Build history of the part. All positions in model axes, mm. A direction names the side the tool comes from. Round coordinates to 2 decimals unless told otherwise and drop trailing zeros. Order: outer loops, then holes, each group sorted by start corner. A loop starts at its lowest first (then second) coordinate and runs counter-clockwise, first axis right, second up. Notation, with made-up numbers: (57, 6) - (100, 6) arc R22 cw to (100, 19) - close; hole circle Ø4 at (23.25, -5.75). An arc over 180 degrees is marked (long way). Write each question's results on one line, items separated by ' | '. Start each with the question number.
```python
from build123d import *

# Parameters (mm, degrees)
F1_DEPTH = 0.889


with BuildPart() as f1:
    # F0 (on Front) → F1 (new body)
    with BuildSketch(Plane.XZ):
        Polygon((-7.766421, 2.049147), (-9.697749, 3.149271), (-8.251928, 3.717801), (-8.401837, 4.58542), (-9.168207, 5.237091), (-10.238115, 4.58542), (-10.238115, 5.944121), (-7.570077, 7.6432), (-7.442288, 8.765532), (-8.34682, 9.053338), (-10.238115, 7.696539), (-10.238115, 10.554039), (-11.1125, 11.030715), (-12.026622, 10.656827), (-12.026622, 7.737654), (-13.897186, 9.053338), (-14.801892, 8.683302), (-14.616874, 7.614309), (-11.972634, 5.904664), (-11.972634, 4.58542), (-13.099057, 5.233018), (-13.897186, 4.58542), (-13.897186, 3.738368), (-12.566103, 3.167905), (-14.415789, 2.044265), (-14.217429, 3.537872), (-15.124985, 3.874964), (-15.949978, 3.513755), (-15.90289, 2.267294), (-17.152183, 2.986197), (-17.271507, 6.144799), (-18.168139, 6.798936), (-18.851348, 6.144799), (-18.678295, 3.910622), (-21.210807, 5.319494), (-21.997354, 4.69717), (-22.072788, 3.808485), (-19.557991, 2.238555), (-21.62216, 1.25008), (-21.850014, 0.367141), (-20.696388, 0), (-18.017134, 1.395444), (-16.867385, 0.695083), (-17.854148, 0.181145), (-17.854148, -0.682273), (-16.887943, -1.360672), (-15.860065, -0.435582), (-15.860065, -2.717471), (-17.038523, -1.745301), (-17.813032, -2.224089), (-17.962941, -3.267605), (-16.876877, -3.790525), (-18.007542, -4.489482), (-20.782813, -3.153241), (-21.790132, -3.523277), (-21.605115, -4.427809), (-19.562521, -5.39587), (-21.992089, -6.886292), (-21.992089, -7.802464), (-21.173319, -8.447639), (-18.651634, -6.953308), (-18.847212, -9.336909), (-18.167692, -9.941154), (-17.27537, -9.146621), (-17.142811, -6.062488), (-15.893939, -5.322416), (-15.948845, -6.659137), (-15.032252, -7.007643), (-14.164055, -6.716586), (-14.440246, -5.05889), (-12.565052, -6.207264), (-13.832696, -6.716586), (-13.832696, -7.661451), (-13.018659, -8.315589), (-11.986575, -7.603306), (-11.986575, -8.984262), (-14.617661, -10.699556), (-14.847309, -11.83401), (-13.893868, -12.164047), (-11.984149, -10.699556), (-11.984149, -13.696965), (-11.1125, -14.067002), (-10.252469, -13.738081), (-10.252469, -10.878737), (-8.323933, -12.14982), (-7.392148, -11.79901), (-7.580517, -10.724198), (-10.252469, -8.963136), (-10.252469, -7.642987), (-9.176794, -8.351956), (-8.370036, -7.740776), (-8.345589, -6.640652), (-9.690185, -6.127262), (-7.661067, -5.051585), (-7.929987, -6.640652), (-7.123229, -6.982913), (-6.292025, -6.640652), (-6.292025, -5.344951), (-4.996324, -6.127262), (-4.800489, -9.098248), (-3.969542, -9.843235), (-3.333915, -9.134266), (-3.505045, -6.934019), (-1.017748, -8.396618), (-0.204675, -7.814118), (-0.204675, -6.860677), (-2.616602, -5.393827), (-0.508032, -4.391492), (-0.355237, -3.444164), (-1.433989, -3.028562), (-4.306216, -4.446499), (-5.440253, -3.713083), (-4.306216, -3.175245), (-4.306216, -2.368488), (-5.126319, -1.7468), (-6.335333, -2.61296), (-6.335333, -0.385276), (-5.125197, -1.31427), (-4.306216, -0.727537), (-4.306216, 0.201456), (-5.345222, 0.739294), (-4.18398, 1.448263), (-1.433989, 0.083229), (-0.370219, 0.411185), (-0.620721, 1.223725), (-2.670654, 2.391408), (-0.225309, 3.809345), (-0.225309, 4.845845), (-1.068589, 5.326194), (-3.684515, 3.809345), (-3.420916, 6.093763), (-4.120606, 6.873983), (-5.028335, 6.059946), (-5.028335, 2.855904), (-6.419651, 2.049147), (-6.419651, 3.41819), (-7.106347, 3.809345), (-7.986446, 3.41819), align=None)
        Polygon((-14.416056, -3.451471), (-14.440504, 0.411185), (-11.115686, 2.391408), (-7.766421, 0.435633), (-7.766421, -3.451471), (-11.017897, -5.431693), align=None, mode=Mode.SUBTRACT)
    extrude(amount=F1_DEPTH)


solid = f1.part
```
1. Wall check: line 1 (Z direction, x = -1.5, y = -0.8); line 2 (Z direction, x = -2, y = -0.2); line 3 (X direction, y = -0.1, z = -0.25). Give the ranges that are in metal, low to high. Write a range as from..to.
2. Cut at B-B (z = -5.75). List the corners of the cut face in (x, y).
3. Cut at A-A (x = -16.25). List the corners of the cut face in (y, z).
4. 3-axis set-ups, long thin cutter, end or side, ignore diameter. For faces 1 (the face through (-1.465, -0.438, 3.09)), 2 (the face through (-14.71, -0.44, 8.16)), 3 (the face through (-13.284, -0.438, -9.83)), 4 (the face through (-15.5, -0.44, -6.83)): which of +Z, -Z, +X, -X, +Y, -Y reach the whole face in a straight line?
5. Mould opens along Z. For faces 5 (the face through (-15.927, -0.438, 2.899)), 6 (the face through (-9.302, -0.438, -11.505)), 7 (the face through (-0.64, -0.44, 5.08)) say: pulls with the +Z half, pulls with the -Z half, needs draft (parallel to the pull), parting line crosses it, or undercut.
A:
1) line 1: z = -8.11..-6.07, -4.86..-3.06, 0.12..1.72, 3.07..5.08 | line 2: z = -7.82..-5.77, -5.1..-3.31, 0.36..2.01, 2.78..4.79 | line 3: x = -17.85..-14.44, -7.77..-4.31
2) outline: (-20.14, -0.89) - (-16.62, -0.89) - (-16.62, 0) - (-20.14, 0) - close; (-15.91, -0.89) - (-14.33, -0.89) - (-14.33, 0) - (-15.91, 0) - close; (-13.31, -0.89) - (-8.98, -0.89) - (-8.98, 0) - (-13.31, 0) - close; (-7.78, -0.89) - (-6.29, -0.89) - (-6.29, 0) - (-7.78, 0) - close; (-5.62, -0.89) - (-2.03, -0.89) - (-2.03, 0) - (-5.62, 0) - close
3) outline: (-0.89, -5.53) - (0, -5.53) - (0, -2.4) - (-0.89, -2.4) - close; (-0.89, -0.79) - (0, -0.79) - (0, 2.47) - (-0.89, 2.47) - close
4) face 1: +X, +Y, -Y | face 2: -X, +Y, -Y | face 3: +Y, -Y | face 4: -Z, +Y, -Y
5) face 5: undercut | face 6: pulls with the -Z half | face 7: pulls with the +Z half
